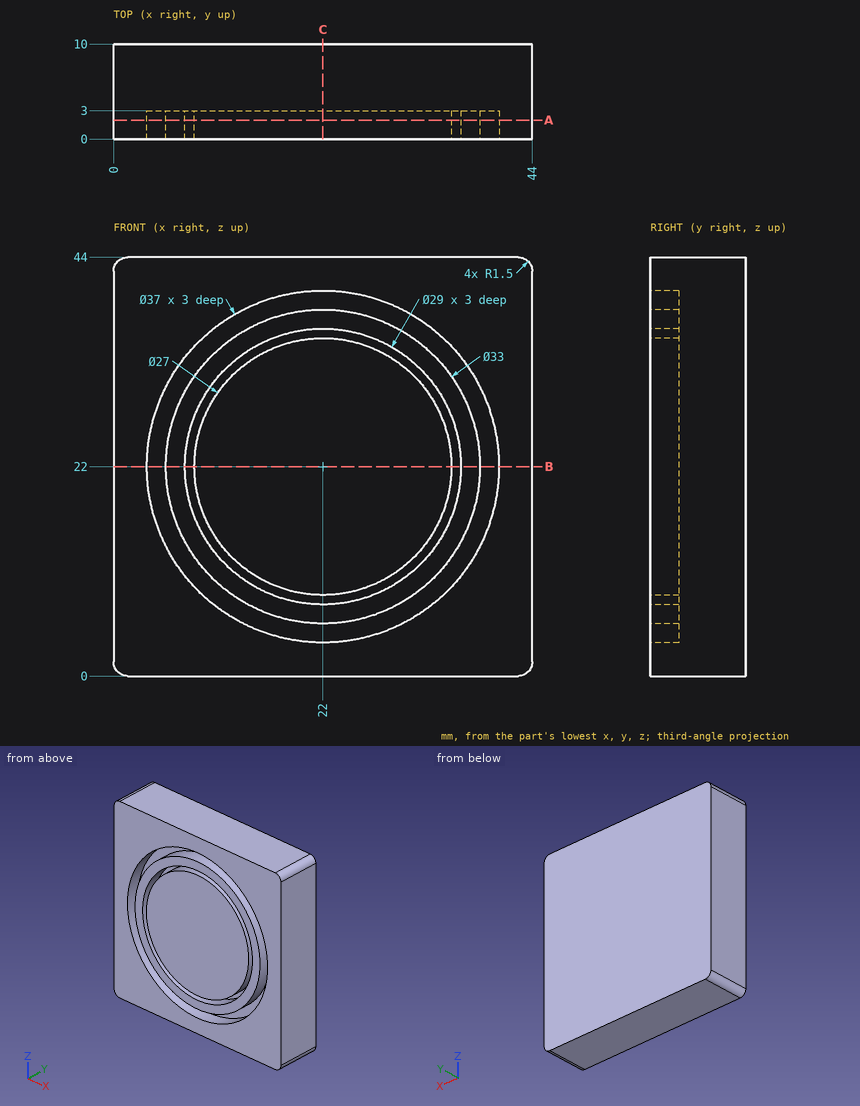
Here's the drawing with two shaded views (mm, measured from the low corner). I have some questions. Round coordinates to 2 decimals unless told otherwise and drop trailing zeros. Order: outer loops, then holes, each group sorted by start corner. A loop starts at its lowest first (then second) coordinate and runs counter-clockwise, first axis right, second up. Notation, with made-up numbers: M 42.25,-26.5 L 47.25,-26.5 A26 ccw 47.25,5.5 Z; hole C 19.5,15 d8. An arc over 180 degrees is marked long. Answer in a Markdown table with one row per item.
Item 1: Imagine slicing it at C-C, the plane x = 22. Write out the boundary of the cut face in (y, z).
A:
| item | result |
|---|---|
| outline | M 0,0 L 10,0 L 10,44 L 0,44 L 0,40.5 L 3,40.5 L 3,38.5 L 0,38.5 L 0,36.5 L 3,36.5 L 3,35.5 L 0,35.5 L 0,8.5 L 3,8.5 L 3,7.5 L 0,7.5 L 0,5.5 L 3,5.5 L 3,3.5 L 0,3.5 Z |
Item 2: Imagine slicing it at B-B, the plane z = 22. Write out the boundary of the cut face in (x, y).
A:
| item | result |
|---|---|
| outline | M 0,0 L 3.5,0 L 3.5,3 L 5.5,3 L 5.5,0 L 7.5,0 L 7.5,3 L 8.5,3 L 8.5,0 L 35.5,0 L 35.5,3 L 36.5,3 L 36.5,0 L 38.5,0 L 38.5,3 L 40.5,3 L 40.5,0 L 44,0 L 44,10 L 0,10 Z |
Item 3: If I drill on L1, parallel to Z at x = 22, y = 1.4; L2, parallel to X at y = 0.75, z = 28; L3, parallel to Z at x = 30, y = 0.5, over which ranges is the centre line in solid material (lowest first)? Write a range as from..to.
A:
| item | result |
|---|---|
| L1 | z = 0..3.5, 5.5..7.5, 8.5..35.5, 36.5..38.5, 40.5..44 |
| L2 | x = 0..4.5, 6.63..8.8, 9.91..34.09, 35.2..37.37, 39.5..44 |
| L3 | z = 0..5.32, 7.57..9.91, 11.13..32.87, 34.09..36.43, 38.68..44 |
Item 4: Imagine slicing it at A-A, the plane y = 2. Write out the boundary of the cut face in (x, z).
A:
| item | result |
|---|---|
| outline | M 0,1.5 A1.5 ccw 1.5,0 L 42.5,0 A1.5 ccw 44,1.5 L 44,42.5 A1.5 ccw 42.5,44 L 1.5,44 A1.5 ccw 0,42.5 Z; C 22,22 d33; C 22,22 d27; hole C 22,22 d37; hole C 22,22 d29 |
Item 5: I'm going to push a flat-ended pin straight in: pin 1 (8.5 mm diameter, centred on x = 29, z = 27.5, fed in from -Y). Where does the tip first touch, or does it pass through?
A:
| item | result |
|---|---|
| pin 1 | stops at y = 0 |
